from build123d import *

# Parameters (mm, degrees)
F0_W          = 84.4335490838
F0_H          = 152.3446664214
F1_DEPTH      = 76.2
F1_DEPTH_BACK = 121.666
F1_TAPER_BACK = -20


with BuildPart() as f1:
    # F0 (on Top) → F1 (new body, two sides)
    with BuildSketch(Plane.XY) as f1_sk:
        with Locations((33.7879988365, -0.1448951662)):
            Rectangle(F0_W, F0_H)
    extrude(amount=F1_DEPTH)
    extrude(f1_sk.sketch, amount=-F1_DEPTH_BACK, taper=F1_TAPER_BACK)


solid = f1.part
Check sheet for the modelled part. Datum: model origin and axes. Units: mm. A direction names the side the tool comes from. Round coordinates to 2 decimals unless told otherwise and drop trailing zeros. Loops run counter-clockwise (first coordinate to the right, second up) from the corner with the lowest first, then second, coordinate; pieces in that order, holes last. Notation, with made-up numbers: (10.5, 66.25) - (57.5, 66.25) arc R21 ccw to (57.5, 93.25) - close; hole circle Ø5 at (-27, 53). An arc over 180 degrees is marked (long way). Answer as CSV lines item,"result". Start each with the question number.
Item 1: Scan lines: line 1 (Y direction, x = 2.5, z = 4.5); line 2 (X direction, y = 21, z = 33); line 3 (Y direction, x = 37, z = -86). Record each from-to range of solid material in increasing order. Write a range as [from, to].
Item 2: Set-up check for faces 1 (the flat face through (76.005, -1, 38)), 2 (the flat face through (33, 1, 76.2)), 3 (the flat face through (-8.429, -1, 38)), 4 (the flat face through (33, 76.027, 38)), 5 (the flat face through (33, -76.317, 38)): record each of +Z, -Z, +X, -X, +Y, -Y from which the full face is reachable in a straight line by a thin tool's end or side.
Item 3: Depth check by flat-ended pin: P1, Ø3, axis at y = 25.5, z = -100.5, coming from the -X side; P2, Ø23, axis at x = 47.5, z = 31.5, coming from the -Y side; P3, Ø5, axis at x = 1.5, z = -25.5, coming from the -Y side. Enter the tip coordinate at first touch or a pass-through.
Item 4: Section check A-A (z = 28). Record the boundary of the cut face in (x, y).
Report:
1,line 1,"y = [-76.32, 76.03]"
1,line 2,"x = [-8.43, 76]"
1,line 3,"y = [-107.62, 107.33]"
2,face 1,"+Z, +X, +Y, -Y"
2,face 2,"+Z, +X, -X, +Y, -Y"
2,face 3,"+Z, -X, +Y, -Y"
2,face 4,"+Z, +X, -X, +Y"
2,face 5,"+Z, +X, -X, -Y"
3,P1,"stops at x = -45.55"
3,P2,"stops at y = -76.32"
3,P3,"stops at y = -86.51"
4,outline,"(-8.43, -76.32) - (76, -76.32) - (76, 76.03) - (-8.43, 76.03) - close"
